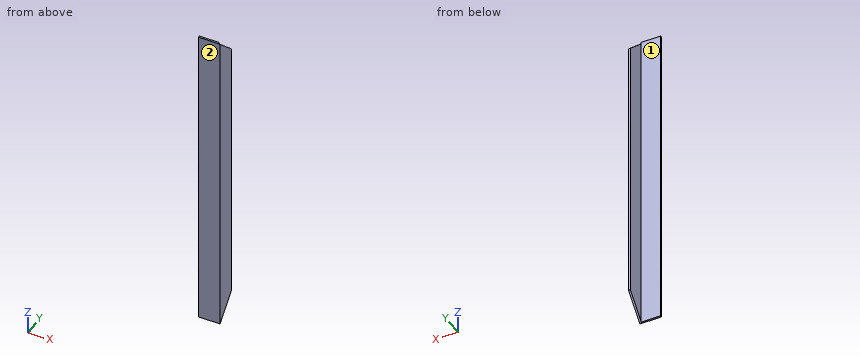
from build123d import *

# Parameters (mm, degrees)
BOSS_EXTRUDE1_DEPTH = 2
SKETCH2_W           = 340
SKETCH2_H           = 2
BOSS_EXTRUDE2_DEPTH = 21.3


with BuildPart() as part:
    # Sketch1 → Boss-Extrude1 (new body)
    with BuildSketch(Plane(origin=(0, 0, 0), x_dir=(0, 0, -1), z_dir=(1, 0, 0))):
        Polygon((-198.982035928, 0), (141.017964072, 0), (116.300201593, 23.3), (-177.018478326, 23.3), align=None)
    extrude(amount=BOSS_EXTRUDE1_DEPTH)

    # Sketch2 → Boss-Extrude2 (add)
    with BuildSketch(Plane.ZY):
        with Locations((28.982035928, 1)):
            Rectangle(SKETCH2_W, SKETCH2_H)
    extrude(amount=BOSS_EXTRUDE2_DEPTH)


solid = part.part
The listing builds one solid part. Answer for the finished solid, in the listing's coordinates (mm). Face numbers are marked on the shaded views. A direction names the side the tool comes from. Give positions to 0.01 mm unless a question says otherwise; leave off trailing zeros. Loops run counter-clockwise (first coordinate to the right, second up) from the corner with the lowest first, then second, coordinate; pieces in that order, holes last.
Item 1: A tool of negligible diameter and unlimited length cuts with its end or side. For the marked faces 1 and 2, from which of +Z, -Z, +X, -X, +Y, -Y can it reach the whole face along a straight path? Write none if from no direction.
Derived:
face 1: +Z, -Z, -X, +Y
face 2: +Z, -Z, +X, -X, -Y
Item 2: A cutting plane is placed at C-C (y = 13). Give the vertices of the cut face in (x, z), then the cut area to 3 significant figures.
Derived:
outline: (0, -127.23) - (2, -127.23) - (2, 186.73) - (0, 186.73) - close
area: 628 mm2
Item 3: Each of these flat-tipped pins is pushed along its axis until it touches: pin 1 Ø6.5 at (y, z) = (7.5, -2) entering from -X; pin 2 Ø10 at (x, y) = (-16.5, 6) entering from -Z; pin 3 Ø10.5 at (x, z) = (-15.5, -43) entering from +Y; pin 4 Ø0.6 at (y, z) = (1.5, -140) entering from +X. Where does it stop, or does it pass through?
Derived:
pin 1: stops at x = 0
pin 2: stops at z = -141.02
pin 3: stops at y = 2
pin 4: stops at x = 0
Item 4: A cutting plane is placed at B-B (x = -8.25). Give the vertices of the cut face in (y, z), then the cut area to 3 significant figures.
Derived:
outline: (0, -141.02) - (2, -141.02) - (2, 198.98) - (0, 198.98) - close
area: 680 mm2
Item 5: A cutting plane is placed at A-A (z = -22). Give the vertices of the cut face in (x, y), then the cut area to 3 significant figures.
Derived:
outline: (-21.3, 0) - (2, 0) - (2, 23.3) - (0, 23.3) - (0, 2) - (-21.3, 2) - close
area: 89.2 mm2
Item 6: Find the intervals of material crossed by line 1 along Y through (x, z) = (-19.25, -117), in increasing order.
Derived:
line 1: y = 0 to 2
